Here's the drawing with two shaded views (mm, measured from the low corner). I have some questions. A direction names the side the tool comes from. Coordinates: 2 decimals unless noted, no trailing zeros. Write each loop counter-clockwise with the first axis right and the second up, starting at its lowest first coordinate (ties: lowest second). Pieces come first, ordered by that corner, then holes. Notation, with made-up numbers: (-33.5, -28) -> (-16.5, -28) arc R29 cw to (-16.5, 1) -> close; hole circle Ø5 at (-12.5, -3.75). An arc over 180 degrees is marked (long way). Put each result on its own line as item: value.
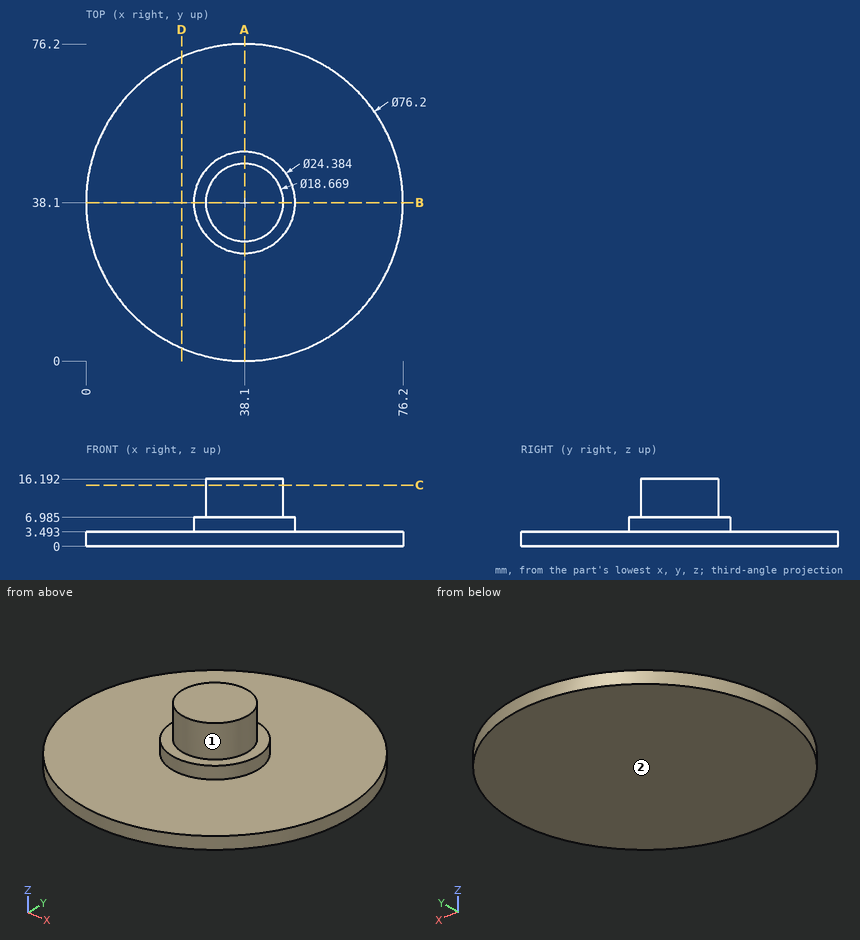
Item 1: Imagine slicing it at D-D on x = 23. Write out the boundary of the cut face in (y, z), then the cut area to 3 significant figures.
Output:
outline: (3.12, 0) -> (73.08, 0) -> (73.08, 3.49) -> (3.12, 3.49) -> close
area: 244 mm²
Item 2: Imagine slicing it at C-C on z = 14.75. Write out the boundary of the cut face in (x, y) (1 decimal), then the cut area to 3 significant figures.
Output:
outline: circle Ø18.7 at (38.1, 38.1)
area: 274 mm²
Item 3: Imagine slicing it at A-A on x = 38.1. Write out the boundary of the cut face in (y, z) (1 decimal).
Output:
outline: (0, 0) -> (76.2, 0) -> (76.2, 3.5) -> (50.3, 3.5) -> (50.3, 7) -> (47.4, 7) -> (47.4, 16.2) -> (28.8, 16.2) -> (28.8, 7) -> (25.9, 7) -> (25.9, 3.5) -> (0, 3.5) -> close
Item 4: Please list where these lines run through material, in increasing order: line 1 along Z through (x, y) = (60.5, 54); line 2 along Y through (x, z) = (41, 4.5); line 3 along Y through (x, z) = (61, 2.25). Write a range as from..to.
Output:
line 1: z = 0..3.49
line 2: y = 26.26..49.94
line 3: y = 7.65..68.55
Item 5: For P1, Ø5, axis at x = 34.5, z = 4, coming from the +Y side; P2, Ø2, axis at x = 68.5, z = 2.5, coming from the -Y side (1 decimal); P3, Ø6, axis at y = 34, z = 10.5, coming from the -X side, each with a flat end and sliding along its axis, tell me the tip position at first contact or that it passes through.
Output:
P1: stops at y = 76.18
P2: stops at y = 13.9
P3: stops at x = 28.83
Item 6: Which directions (+Z, -Z, +X, -X, +Y, -Y) give clear straight access to the entire face, cutting with the end or side of a thin tool? Please do the marked faces 1 and 2.
Output:
face 1: +Z
face 2: -Z, +X, -X, +Y, -Y
